```python
from build123d import *

# Parameters (mm, degrees)
SKETCH1_R           = 5
SKETCH1_R_2         = 2
SKETCH1_R_3         = 4
SKETCH1_R_4         = 1.5
BOSS_EXTRUDE1_DEPTH = 5


with BuildPart() as part:
    # Sketch1 → Boss-Extrude1 (new body)
    with BuildSketch(Plane(origin=(0, 0, 0), x_dir=(1, 0, 0), z_dir=(0, 1, 0))):
        with BuildLine():
            ThreePointArc((4.164387077, 20.582951204), (-20.032105437, 6.301964119), (-8.369909934, -19.259922318))
            ThreePointArc((-8.369909934, -19.259922318), (99.738576714, -39.831721611), (206.206468023, -11.98873449))
            ThreePointArc((206.206468023, -11.98873449), (212.890441324, 4.010800728), (198.30885544, 13.393656337))
            ThreePointArc((198.30885544, 13.393656337), (100.943706101, 9.078229318), (4.164387077, 20.582951204))
        make_face()
        Circle(SKETCH1_R, mode=Mode.SUBTRACT)
        with Locations((0, 12)):
            Circle(SKETCH1_R_2, mode=Mode.SUBTRACT)
        with Locations((12, 0)):
            Circle(SKETCH1_R_2, mode=Mode.SUBTRACT)
        with Locations((0, -12)):
            Circle(SKETCH1_R_2, mode=Mode.SUBTRACT)
        with Locations((-12, 0)):
            Circle(SKETCH1_R_2, mode=Mode.SUBTRACT)
        with Locations((200, 0)):
            Circle(SKETCH1_R_3, mode=Mode.SUBTRACT)
        with Locations((50, 0)):
            Circle(SKETCH1_R_4, mode=Mode.SUBTRACT)
        with Locations((150, 0)):
            Circle(SKETCH1_R_4, mode=Mode.SUBTRACT)
        with BuildLine():
            ThreePointArc((151.229508397, -25.872674783), (155.897333295, -18.894803181), (149.019607843, -14.08063929))
            ThreePointArc((149.019607843, -14.08063929), (100, -18.112603774), (50.980392157, -14.08063929))
            ThreePointArc((50.980392157, -14.08063929), (44.102666705, -18.894803181), (48.770491603, -25.872674783))
            ThreePointArc((48.770491603, -25.872674783), (100, -31.177890471), (151.229508397, -25.872674783))
        make_face(mode=Mode.SUBTRACT)
    extrude(amount=BOSS_EXTRUDE1_DEPTH)


solid = part.part
```
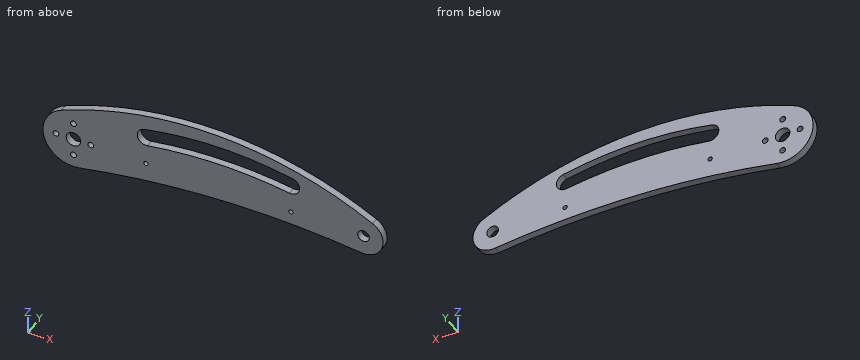
Build history of the part. All positions in model axes, mm. Coordinates: 2 decimals unless noted, no trailing zeros. Write each loop counter-clockwise with the first axis right and the second up, starting at its lowest first coordinate (ties: lowest second). Pieces come first, ordered by that corner, then holes.
1. Drill centre lines: probe 1 along Z at (x, y) = (150, 1.85); probe 2 along X at (y, z) = (3.7, -2.5); probe 3 along Z at (x, y) = (109.5, 0.65). Where is each one in solid material? Low to high.
Answer block:
probe 1: z = -9.27 to -1.5, 1.5 to 14, 26.13 to 32.98
probe 2: x = -20.85 to -4.33, 4.33 to 196.88, 203.12 to 213.27
probe 3: z = -8.82 to 17.96, 31 to 39.31
2. Band-saw the part on A-A, the plane z = 22. Give the cut face in (x, y).
Answer block:
outline: (-1.81, 0) - (44.34, 0) - (44.34, 5) - (-1.81, 5) - close; (155.66, 0) - (184.35, 0) - (184.35, 5) - (155.66, 5) - close
3. Band-saw the part on D-D, the plane x = 32.5. Give the cut face in (y, z).
Answer block:
outline: (0, -15.55) - (5, -15.55) - (5, 32.97) - (0, 32.97) - close
4. Band-saw the part on B-B, the plane x = 118. Give the cut face in (y, z), and give its area (3 significant figures).
Answer block:
outline: (0, -8.69) - (5, -8.69) - (5, 17.57) - (0, 17.57) - close; (0, 30.53) - (5, 30.53) - (5, 38.54) - (0, 38.54) - close
area: 171 mm2
5. Band-saw the part on C-C, the plane y = 0.95. Give the number of separate pieces and of enclosed holes in the cut face, and give its area (3 significant figures).
Answer block:
separate pieces: 1
enclosed holes: 9
area: 8,380 mm2
6. Drop flat-ended pins along their axis: pin 1 (1 mm diameter, centred on x = 133, y = 1, fed in from +Z); pin 2 (5 mm diameter, centred on x = 200, z = 0, fed in from +Y); pin 3 (5 mm diameter, centred on x = 12, z = 0, fed in from +Y); pin 4 (2 mm diameter, centred on x = 107, y = 3, fed in from -Z). Give the stop position or say it passes through.
Answer block:
pin 1: stops at z = 36.55
pin 2: passes through
pin 3: stops at y = 5
pin 4: stops at z = -8.91
